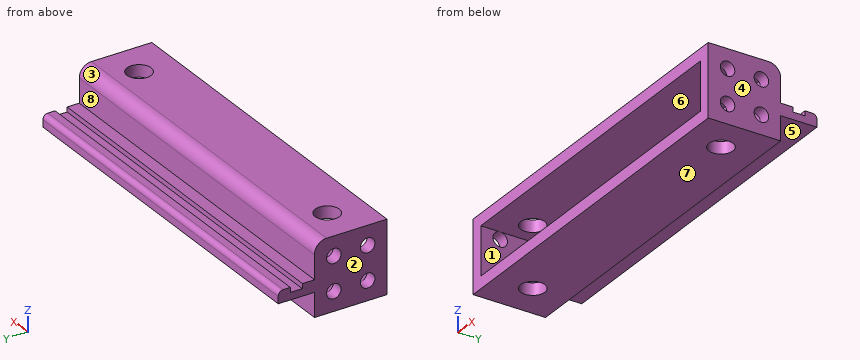
```python
from build123d import *

# Parameters (mm, degrees)
SKETCH2_W               = 150
SKETCH2_H               = 30
BOSS_EXTRUDE1_DEPTH     = 30
SHELL1_T                = -5
CUT_EXTRUDE1_DEPTH      = 156.884572681
CUT_EXTRUDE1_DEPTH_BACK = 156.884572681
SKETCH3_R               = 3
CUT_EXTRUDE2_DEPTH      = 156.884572681
CUT_EXTRUDE2_DEPTH_BACK = 156.884572681
SKETCH5_R               = 5
SKETCH6_W               = 150
SKETCH6_H               = 5
BOSS_EXTRUDE3_DEPTH     = 15
SKETCH7_W               = 150
SKETCH7_H               = 5
CUT_EXTRUDE3_DEPTH      = 2
FILLET1_R               = 2
FILLET2_R               = 5


with BuildPart() as part:
    # Sketch2 → Boss-Extrude1 (new body)
    with BuildSketch(Plane(origin=(0, 0, 0), x_dir=(1, 0, 0), z_dir=(0, 1, 0))):
        with Locations((-75, 15)):
            Rectangle(SKETCH2_W, SKETCH2_H)
    extrude(amount=BOSS_EXTRUDE1_DEPTH)

    # Shell1
    shell1_openings = [part.faces().sort_by_distance(p)[0] for p in [
        (-75, 0, -15),
    ]]
    offset(amount=SHELL1_T, openings=shell1_openings, kind=Kind.INTERSECTION)

    # Sketch3 → Cut-Extrude1 (cut, two sides: drawn at the far end of the back side and taken through both)
    with BuildSketch(Plane.ZY.offset(150).offset(-CUT_EXTRUDE1_DEPTH_BACK)):
        with Locations(Location((-22, 22, 0), (0, 0, 180))):
            Circle(SKETCH3_R)
        with Locations((-8, 22)):
            Circle(SKETCH3_R)
        with Locations((-8, 8)):
            Circle(SKETCH3_R)
        with Locations(Location((-22, 8, 0), (0, 0, 180))):
            Circle(SKETCH3_R)
    extrude(amount=CUT_EXTRUDE1_DEPTH + CUT_EXTRUDE1_DEPTH_BACK, mode=Mode.SUBTRACT)

    # Sketch5 → Cut-Extrude2 (cut, two sides: drawn at the far end of the back side and taken through both)
    with BuildSketch(Plane.XY.offset(-CUT_EXTRUDE2_DEPTH_BACK)):
        with Locations(Location((-135, 15, 0), (0, 0, 180))):
            Circle(SKETCH5_R)
        with Locations(Location((-15, 15, 0), (0, 0, 180))):
            Circle(SKETCH5_R)
    extrude(amount=CUT_EXTRUDE2_DEPTH + CUT_EXTRUDE2_DEPTH_BACK, mode=Mode.SUBTRACT)

    # Sketch6 → Boss-Extrude3 (add)
    with BuildSketch(Plane(origin=(0, 30, 0), x_dir=(1, 0, 0), z_dir=(0, 1, 0))):
        with Locations((-75, 17.5)):
            Rectangle(SKETCH6_W, SKETCH6_H)
    extrude(amount=BOSS_EXTRUDE3_DEPTH)

    # Sketch7 → Cut-Extrude3 (cut)
    with BuildSketch(Plane.XY.offset(-15)):
        with Locations((-75, 37.5)):
            Rectangle(SKETCH7_W, SKETCH7_H)
    extrude(amount=-CUT_EXTRUDE3_DEPTH, mode=Mode.SUBTRACT)

    # Fillet1
    fillet1_edges = [part.edges().sort_by_distance(p)[0] for p in [
        (-75, 45, -15),
    ]]
    fillet(fillet1_edges, radius=FILLET1_R)

    # Fillet2
    fillet2_edges = [part.edges().sort_by_distance(p)[0] for p in [
        (-75, 30, 0),
    ]]
    fillet(fillet2_edges, radius=FILLET2_R)


solid = part.part
```
Geometry check sheet. Reference: the model listing, model coordinates, mm. Face numbers are marked on the shaded views. A direction names the side the tool comes from. Coordinates: 2 decimals unless noted, no trailing zeros. Order: outer loops, then holes, each group sorted by start corner. A loop starts at its lowest first (then second) coordinate and runs counter-clockwise, first axis right, second up. Notation, with made-up numbers: M 81,-17 L 86,-17 A25 ccw 86,22 Z; hole C 37.5,-23.5 d2. An arc over 180 degrees is marked long. One line per question, with ' | ' between items. Start each with the question number.
Item 1: Draft check along X on the marked faces 1, 2, 3 and 4. Enter one of: pulls with the +X half, pulls with the -X half, needs draft (parallel to the pull), parting line crosses it, or undercut.
Item 2: Cross-section at D-D on x = -105. Enter the section's corners in (y, z).
Item 3: Material ranges on L1, parallel to Z at x = -2.35, y = 22; L2, parallel to Y at x = -148, z = -22; L3, parallel to Z at x = -122, y = 23, recorded low to high. Write a range as [from, to].
Item 4: Set-up check for the marked faces 5, 6, 7 and 8: record each of +Z, -Z, +X, -X, +Y, -Y from which the full face is reachable in a straight line by a thin tool's end or side.
Item 5: Cross-section at B-B on y = 15. Enter the section's corners in (x, z), then the cut area to 3 significant figures.
Item 6: Gauge pin test, flat ends, axial feed: pin 1 (7.5 mm diameter, centred on x = -90.5, y = 34, fed in from -Z); pin 2 (4 mm diameter, centred on x = -109, z = -3, fed in from +Y); pin 3 (0.6 mm diameter, centred on x = -60, z = -16.5, fed in from -Y). Record the tip position at first contact, or that the pin passes through.
Item 7: Cross-section at A-A on x = -135. Enter the section's corners in (y, z).
Item 8: Cross-section at C-C on z = -6.5. Enter the section's corners in (x, y), then the cut area to 3 significant figures.
Findings:
1) face 1: undercut | face 2: pulls with the -X half | face 3: needs draft | face 4: pulls with the +X half
2) outline: M 0,-30 L 30,-30 L 30,-20 L 45,-20 L 45,-17 A2 ccw 43,-15 L 40,-15 L 40,-17 L 35,-17 L 35,-15 L 30,-15 L 30,-5 A5 ccw 25,0 L 0,0 L 0,-5 L 25,-5 L 25,-25 L 0,-25 Z
3) L1: z = [-30, -25], [-19, -11], [-5, 0] | L2: y = [0, 5], [11, 19], [25, 30] | L3: z = [-30, -25], [-5, 0]
4) face 5: -Z, +X, -X, +Y | face 6: -Y | face 7: -Z, +X, -X, +Y, -Y | face 8: +Z, +X, -X, +Y
5) outline: M -150,-30 L -140,-30 L -140,-25 L -145,-25 L -145,-5 L -140,-5 L -140,0 L -150,0 Z; M -130,-30 L -20,-30 L -20,-25 L -130,-25 Z; M -130,-5 L -20,-5 L -20,0 L -130,0 Z; M -10,-30 L 0,-30 L 0,0 L -10,0 L -10,-5 L -5,-5 L -5,-25 L -10,-25 Z | area: 1,500 mm²
6) pin 1: stops at z = -20 | pin 2: stops at y = 30 | pin 3: stops at y = 25
7) outline: M 0,-30 L 10,-30 L 10,-25 L 0,-25 Z; M 0,-5 L 10,-5 L 10,0 L 0,0 Z; M 20,-30 L 30,-30 L 30,-20 L 45,-20 L 45,-17 A2 ccw 43,-15 L 40,-15 L 40,-17 L 35,-17 L 35,-15 L 30,-15 L 30,-5 A5 ccw 25,0 L 20,0 L 20,-5 L 25,-5 L 25,-25 L 20,-25 Z
8) outline: M -150,0 L -145,0 L -145,5.4 L -150,5.4 Z; M -150,10.6 L -145,10.6 L -145,19.4 L -150,19.4 Z; M -150,24.6 L -145,24.6 L -145,25 L -5,25 L -5,24.6 L 0,24.6 L 0,30 L -150,30 Z; M -5,0 L 0,0 L 0,5.4 L -5,5.4 Z; M -5,10.6 L 0,10.6 L 0,19.4 L -5,19.4 Z | area: 896 mm²
